Verification items for the finished model (mm, model axes). A direction names the side the tool comes from. Give positions to 0.01 mm unless a question says otherwise; leave off trailing zeros. Order: outer loops, then holes, each group sorted by start corner. A loop starts at its lowest first (then second) coordinate and runs counter-clockwise, first axis right, second up.
(1) Sectioned sample at A-A on y = 4. Count the separate pieces of the cut face and the enclosed holes in it, plus the area to 3 significant figures.
(2) Sectioned sample at B-B on x = -2.5. Record the cut outline in (y, z).
(3) Mould release check, pull along Z, two halves, no side actions. Record for faces 4 (the face through (-17, 4.762, 5)), 5 (the face through (17.888, 4, 0)), 6 (the face through (0, 4, 22.838)), 7 (the face through (4.67, 3.15, -17.01)): pulls with the +Z half, pulls with the -Z half, needs draft (parallel to the pull), parting line crosses it, or undercut.
(4) Scan lines: L1, parallel to Z at x = 12.1, y = 2.25; L2, parallel to Z at x = -12.1, y = 3.45; L3, parallel to Z at x = 8, y = 1.75. Record each from-to range of solid material in increasing order.
(5) Access from +Z, -Z, +X, -X, +Y, -Y to the whole of each face (thin tool, end or side, straight path). Record for faces 1 (the face through (0, 5, 21.25)), 2 (the face through (-17.888, 4, 0)), 3 (the face through (-17, 6, -1.95)).
(6) Gauge pin test, flat ends, axial feed: pin 1 (5.5 mm diameter, centred on x = -12.1, z = 17.05, fed in from +Y); pin 2 (3 mm diameter, centred on x = -12.1, z = -17.15, fed in from -Y); pin 3 (10 mm diameter, centred on x = -6, z = -1, fed in from +Y). Record the tip position at first contact, or that the pin passes through.
Autodesk Inventor part; units mm, degrees
ref_plane "YZ Plane" through (0, 0, 0) normal (1, 0, 0) x (0, 1, 0)
ref_plane "XZ Plane" through (0, 0, 0) normal (0, 1, 0) x (-1, 0, 0)
ref_plane "XY Plane" through (0, 0, 0) normal (0, 0, 1) x (1, 0, 0)
sketch "Sketch1" plane through (0, 0, 0) normal (0, 1, 0) x (-1, 0, 0)
  line L0 (16.3, 21.25) -> (-16.3, 21.25)
  line L1 (-16.3, 21.25) -> (-16.3, -21.25)
  line L2 (-16.3, -21.25) -> (16.3, -21.25)
  line L3 (16.3, -21.25) -> (16.3, 21.25)
  line L4 (16.3, 21.25) -> (-16.3, -21.25) construction
  line L5 (-16.3, 21.25) -> (16.3, -21.25) construction
  circle A0 centre (12.1, 17.05) radius 1.7
  circle A1 centre (12.1, -17.15) radius 1.7
  circle A2 centre (-12.1, 17.05) radius 1.7
  point P0 (0, 0)
  dimension "d0" = 42.5
  dimension "d1" = 32.6
  dimension "d4" = 3.4
  dimension "d5" = 3.4
  dimension "d6" = 3.4
  dimension "d7" = 34.2
  dimension "d8" = 24.2
  dimension "d9" = 4.2
  dimension "d10" = 4.2
  dimension "d11" = 4.2
  dimension "d12" = 4.2
extrude "Extrusion1" add sketch "Sketch1" along normal blind 1.5875
sketch "Sketch2" plane through (0, 1.5875, 0) normal (0, 1, 0) x (1, 0, 0)
  circle A0 centre (-12.1, -17.05) radius 1.7
  circle A1 centre (-12.1, -17.05) radius 1.7
  circle A2 centre (-12.1, -17.05) radius 3.2875
  circle A3 centre (12.1, -17.05) radius 1.7
  circle A4 centre (12.1, -17.05) radius 1.7
  circle A5 centre (12.1, -17.05) radius 3.2875
  circle A6 centre (-12.1, 17.15) radius 1.7
  circle A7 centre (-12.1, 17.15) radius 1.7
  circle A8 centre (-12.1, 17.15) radius 3.2875
  line L0 (16.3, 21.25) -> (-16.3, 21.25) construction
  line L1 (0, 21.25) -> (0, -21.2058) construction
  circle A9 centre (7.9542, 17.15) radius 3.2875
  point P0 (0, 0)
  dimension "d13" = 1.5875
  dimension "d14" = 1.5875
  dimension "d15" = 1.5875
  dimension "d28" = 6.575
  dimension "d29" = 6.575
extrude "Extrusion2" add sketch "Sketch2" along normal blind 3.175
sketch "Sketch3" plane through (0, 0, 0) normal (0, -1, 0) x (1, 0, 0)
  line L0 (17.8875, 22.8375) -> (-17.8875, 22.8375)
  line L1 (-17.8875, 22.8375) -> (-17.8875, -22.8375)
  line L2 (-17.8875, -22.8375) -> (17.8875, -22.8375)
  line L3 (17.8875, -22.8375) -> (17.8875, 22.8375)
  line L4 (17.8875, 22.8375) -> (-17.8875, -22.8375) construction
  line L5 (-17.8875, 22.8375) -> (17.8875, -22.8375) construction
  line L6 (16.3, -21.25) -> (-16.3, -21.25)
  line L7 (16.3, 21.25) -> (16.3, -21.25)
  line L8 (-16.3, 21.25) -> (16.3, 21.25)
  line L9 (16.3, 21.25) -> (16.3, -21.25)
  line L10 (16.3, -21.25) -> (-16.3, -21.25)
  line L11 (-16.3, -21.25) -> (-16.3, 21.25)
  line L12 (-16.3, 21.25) -> (16.3, -21.25) construction
  line L13 (16.3, 21.25) -> (-16.3, -21.25) construction
  point P0 (0, 0)
  point P1 (-16.3, -21.25)
  dimension "d18" = 1.5875
  dimension "d19" = 1.5875
  dimension "d26" = 35.775
  dimension "d27" = 45.675
extrude "Extrusion3" add sketch "Sketch3" against normal blind 7.9625
sketch "Sketch4" plane through (0, 7.9625, 0) normal (0, 1, 0) x (1, 0, 0)
  line L0 (-16.3, 21.25) -> (-16.3, -21.25)
  line L1 (-17.8875, -22.8375) -> (-17.8875, 22.8375)
  line L2 (-16.3, -12.05) -> (-17.8875, -12.05)
  line L3 (-17.8875, -12.05) -> (-17.8875, 1.95)
  line L4 (-17.8875, 1.95) -> (-16.3, 1.95)
  line L5 (-16.3, 1.95) -> (-16.3, -12.05)
  circle A0 centre (-12.1, -17.05) radius 1.7 construction
  circle A1 centre (-12.1, -17.05) radius 1.7 construction
  point P0 (0, 0)
  point P1 (-17.0938, -12.05)
  point P2 (-17.0938, 1.95)
  dimension "d22" = 5
  dimension "d23" = 14
extrude "Extrusion4" cut sketch "Sketch4" against normal blind 3.2
equation "\"d4\" = m3_clearance"
equation "\"d5\" = m3_clearance"
equation "\"d6\" = m3_clearance"
equation "\"d10\" = d9"
equation "\"d11\" = d9"
equation "\"d12\" = d9"
equation "\"d14\" = d13"
equation "\"d15\" = d13"
equation "\"d29\" = d28"
equation "\"m3_heat_set_insert\" = 4"
equation "\"m3_clearance\" = 3.4"
equation "\"m3_heat_set_depth\" = 7"
equation "\"robot_diameter\" = 354"
equation "\"hardboard_thickness\" = 5"
equation "\"motor_centerline_height\" = 13"
properties part number "microphone_MCU_case"
Ans:
1. separate pieces: 5
1. enclosed holes: 4
1. area: 357 mm2
2. outline: (0, -22.84) - (7.96, -22.84) - (7.96, -21.25) - (1.59, -21.25) - (1.59, 21.25) - (7.96, 21.25) - (7.96, 22.84) - (0, 22.84) - close
3. face 4: undercut
3. face 5: needs draft
3. face 6: pulls with the +Z half
3. face 7: undercut
4. L1: z = -22.84 to -21.25, 13.76 to 15.35, 18.75 to 20.34, 21.25 to 22.84
4. L2: z = -22.84 to -21.25, -20.44 to -18.85, -15.45 to -13.86, 13.76 to 15.35, 18.75 to 20.34, 21.25 to 22.84
4. L3: z = -22.84 to -21.25, -20.44 to -13.86, 21.25 to 22.84
5. face 1: +Y
5. face 2: +Z, -Z, -X, +Y, -Y
5. face 3: -X, +Y
6. pin 1: stops at y = 4.76
6. pin 2: passes through
6. pin 3: stops at y = 1.59
